Geometry: final body of the model. Coordinates: model frame, mm. A direction names the side the tool comes from. Give positions to 0.01 mm unless a question says otherwise; leave off trailing zeros. Loops run counter-clockwise (first coordinate to the right, second up) from the corner with the lowest first, then second, coordinate; pieces in that order, holes last. Notation, with made-up numbers: (8.25, 71.25) - (36.25, 71.25) arc R17 cw to (36.25, 101.25) - close; hole circle Ø3 at (18, 65.5). An arc over 180 degrees is marked (long way). Use CSV: the item, a comma, the result in double quotes. Start each with the question number.
```python
from build123d import *


with BuildPart() as part:
    # Esboço1 → Revolução1 (revolve)
    with BuildSketch(Plane.XY, mode=Mode.PRIVATE) as revolu_o1_sk:
        Polygon((2.1, 0), (8.15, 0), (8.15, -13.3), (1.5, -13.3), (1.5, -15.3), (1.7, -15.3), (1.5, -15.8), (1.5, -17.3), (1.7, -17.3), (1.5, -17.8), (1.5, -19.3), (1.7, -19.3), (1.5, -19.8), (1.5, -21.3), (1.7, -21.3), (1.5, -21.8), (1.5, -23.3), (1, -23.3), (1.25, 0), (0.5, 12), (1.4, 12), align=None)
    revolve(revolu_o1_sk.sketch.rotate(Axis((0, 23.058079528, 0), (0, -1, 0)), 90), axis=Axis((0, 23.058079528, 0), (0, -1, 0)))

    # Esboço2 → Revolução2 (revolve)
    with BuildSketch(Plane.XY, mode=Mode.PRIVATE) as revolu_o2_sk:
        Polygon((1.5, -14.8), (2.5, -13.3), (1.5, -13.3), align=None)
        Polygon((2.1, 0), (2.041765662, 0.998302941), (3.1, 0), align=None)
    revolve(revolu_o2_sk.sketch.rotate(Axis((0, 0.658037097, 0), (0, -1, 0)), 270), axis=Axis((0, 0.658037097, 0), (0, -1, 0)))


solid = part.part
```
Item 1: Pin query (flat end, axial travel): pin 1 Ø4 at (x, z) = (6, 0) entering from +Y; pin 2 Ø2 at (x, y) = (-2.5, -12) entering from -Z; pin 3 Ø1 at (y, z) = (-3, -6) entering from -X. Return the tip coordinate at first contact, or that it passes through.
Item 2: Reachability of faces 1 (the cylindrical face through (4.959, -6.743, -6.468)), 2 (the cylindrical face through (-0.45, -18.56, 1.43)) from +Z, -Z, +X, -X, +Y, -Y: full face, straight path, thin tool, end or side. Return the list, or none.
Item 3: Section C-C (x = 5.5). Output: boundary loops of the cut face in (y, z).
Item 4: Ray query, probe 1 along X at (y, z) = (-4, 0.5); probe 2 along Y at (x, z) = (-6.75, -2.75); probe 3 along Z at (x, y) = (0.75, -3). Return the intervals inside material, ascending.
Item 5: Mould query, pull axis Y, two halves, no side actions, for faces 3 (the flat face through (0, 0, -4)), 4 (the cylindrical face through (-0.45, -15.05, 1.43)), 5 (the conical face through (-0.338, -11.487, 1.075)), 6 (the cylindrical face through (-0.45, -22.56, 1.43)). Classes: pulls with the +Y half, pulls with the -Y half, needs draft (parallel to the pull), parting line crosses it, or undercut.
Item 6: Section B-B (z = -3.5). Output: boundary loops of the cut face in (x, y).
Item 7: Section A-A (y = 3.5). Output: boundary loops of the cut face in (x, z).
Outcome:
1,pin 1,"stops at y = 0"
1,pin 2,"stops at z = -8.01"
1,pin 3,"stops at x = -6.01"
2,face 1,"+Y, -Y"
2,face 2,"none"
3,outline,"(-13.3, -6.01) - (0, -6.01) - (0, 6.01) - (-13.3, 6.01) - close"
4,probe 1,"x = -8.13 to -1.1, 1.1 to 8.13"
4,probe 2,"y = -13.3 to 0"
4,probe 3,"z = -8.12 to -0.96, 0.96 to 8.12"
5,face 3,"pulls with the +Y half"
5,face 4,"undercut"
5,face 5,"undercut"
5,face 6,"needs draft"
6,outline,"(-7.36, -13.3) - (7.36, -13.3) - (7.36, 0) - (-7.36, 0) - close"
7,outline,"circle Ø3.79 at (0, 0); hole circle Ø2.06 at (0, 0)"
